from build123d import *

# Parameters (mm, degrees)
SKETCH1_W                      = 60
SKETCH1_H                      = 430.5
BASE_FLANGE1_DEPTH             = 4
EDGE_FLANGE1_STRIP_W           = 18
EDGE_FLANGE1_STRIP_H           = 4
EDGE_FLANGE1_STRIP_CUT_DEPTH   = 430.5
EDGE_FLANGE1_DEPTH             = 430.5
EDGE_FLANGE2_STRIP_W           = 18
EDGE_FLANGE2_STRIP_H           = 4
EDGE_FLANGE2_STRIP_CUT_DEPTH   = 55
EDGE_FLANGE2_STRIP_2_W         = 18
EDGE_FLANGE2_STRIP_2_H         = 4
EDGE_FLANGE2_STRIP_CUT_2_DEPTH = 55
EDGE_FLANGE2_STRIP_3_W         = 18
EDGE_FLANGE2_STRIP_3_H         = 4
EDGE_FLANGE2_STRIP_CUT_3_DEPTH = 55
EDGE_FLANGE2_STRIP_4_W         = 18
EDGE_FLANGE2_STRIP_4_H         = 4
EDGE_FLANGE2_STRIP_CUT_4_DEPTH = 55
EDGE_FLANGE2_DEPTH             = 55
EDGE_FLANGE2_BEND_DEPTH        = 55
EDGE_FLANGE2_BEND_2_DEPTH      = 55
EDGE_FLANGE2_BEND_3_DEPTH      = 55
SKETCH18_R                     = 4.6
EXTRUDE1_DEPTH                 = 440.643321341
SKETCH19_R                     = 4.6
EXTRUDE2_DEPTH                 = 4
SKETCH20_R                     = 4.6
EXTRUDE3_DEPTH                 = 4


# Sheet-metal steps are written as plain solids
with BuildPart() as part:
    # Sketch1 → Base-Flange1 (new body)
    with BuildSketch(Plane(origin=(0, 0, 0), x_dir=(1, 0, 0), z_dir=(0, 1, 0))):
        Rectangle(SKETCH1_W, SKETCH1_H)
    extrude(amount=BASE_FLANGE1_DEPTH)

    # Edge-Flange1 strip (across the edge) → Edge-Flange1 strip cut (cut)
    with BuildSketch(Plane(origin=(-30, 4, -215.25), x_dir=(1, 0, 0), z_dir=(0, 0, 1))):
        with Locations((-4, -2)):
            Rectangle(EDGE_FLANGE1_STRIP_W, EDGE_FLANGE1_STRIP_H)
    extrude(amount=EDGE_FLANGE1_STRIP_CUT_DEPTH, mode=Mode.SUBTRACT)

    # Edge-Flange1 section (across the edge) → Edge-Flange1 (add)
    with BuildSketch(Plane(origin=(-30, 4, -215.25), x_dir=(1, 0, 0), z_dir=(0, 0, 1))):
        with BuildLine():
            Line((0, 1), (0, 56))
            Line((0, 56), (4, 56))
            Line((4, 56), (4, 1))
            ThreePointArc((4, 1), (4.292893219, 0.292893219), (5, 0))
            Line((5, 0), (5, -4))
            ThreePointArc((5, -4), (1.464466094, -2.535533906), (0, 1))
        make_face()
    extrude(amount=EDGE_FLANGE1_DEPTH)

    # Edge-Flange2 strip (across the edge) → Edge-Flange2 strip cut (cut)
    with BuildSketch(Plane(origin=(-30, 5, 215.25), x_dir=(0, 0, -1), z_dir=(0, 1, 0))):
        with Locations((-4, -2)):
            Rectangle(EDGE_FLANGE2_STRIP_W, EDGE_FLANGE2_STRIP_H)
    extrude(amount=EDGE_FLANGE2_STRIP_CUT_DEPTH, mode=Mode.SUBTRACT)

    # Edge-Flange2 strip 2 (across the edge) → Edge-Flange2 strip cut 2 (cut)
    with BuildSketch(Plane(origin=(30, 0, 215.25), x_dir=(0, 0, -1), z_dir=(-1, 0, 0))):
        with Locations((-4, -2)):
            Rectangle(EDGE_FLANGE2_STRIP_2_W, EDGE_FLANGE2_STRIP_2_H)
    extrude(amount=EDGE_FLANGE2_STRIP_CUT_2_DEPTH, mode=Mode.SUBTRACT)

    # Edge-Flange2 strip 3 (across the edge) → Edge-Flange2 strip cut 3 (cut)
    with BuildSketch(Plane(origin=(-30, 60, -215.25), x_dir=(0, 0, 1), z_dir=(0, -1, 0))):
        with Locations((-4, -2)):
            Rectangle(EDGE_FLANGE2_STRIP_3_W, EDGE_FLANGE2_STRIP_3_H)
    extrude(amount=EDGE_FLANGE2_STRIP_CUT_3_DEPTH, mode=Mode.SUBTRACT)

    # Edge-Flange2 strip 4 (across the edge) → Edge-Flange2 strip cut 4 (cut)
    with BuildSketch(Plane(origin=(-25, 0, -215.25), x_dir=(0, 0, 1), z_dir=(1, 0, 0))):
        with Locations((-4, -2)):
            Rectangle(EDGE_FLANGE2_STRIP_4_W, EDGE_FLANGE2_STRIP_4_H)
    extrude(amount=EDGE_FLANGE2_STRIP_CUT_4_DEPTH, mode=Mode.SUBTRACT)

    # Edge-Flange2 section (across the edge) → Edge-Flange2 (add)
    with BuildSketch(Plane(origin=(-30, 5, 215.25), x_dir=(0, 0, -1), z_dir=(0, 1, 0))):
        with BuildLine():
            Line((0, 1), (0, 36))
            Line((0, 36), (4, 36))
            Line((4, 36), (4, 1))
            ThreePointArc((4, 1), (4.292893219, 0.292893219), (5, 0))
            Line((5, 0), (5, -4))
            ThreePointArc((5, -4), (1.464466094, -2.535533906), (0, 1))
        make_face()
    extrude(amount=EDGE_FLANGE2_DEPTH)

    # Edge-Flange2 section 2 (across the edge) → Edge-Flange2 bend (add)
    with BuildSketch(Plane(origin=(30, 0, 215.25), x_dir=(0, 0, -1), z_dir=(-1, 0, 0))):
        with BuildLine():
            Line((0, 1), (0, 36))
            Line((0, 36), (4, 36))
            Line((4, 36), (4, 1))
            ThreePointArc((4, 1), (4.292893219, 0.292893219), (5, 0))
            Line((5, 0), (5, -4))
            ThreePointArc((5, -4), (1.464466094, -2.535533906), (0, 1))
        make_face()
    extrude(amount=EDGE_FLANGE2_BEND_DEPTH)

    # Edge-Flange2 section 3 (across the edge) → Edge-Flange2 bend 2 (add)
    with BuildSketch(Plane(origin=(-30, 60, -215.25), x_dir=(0, 0, 1), z_dir=(0, -1, 0))):
        with BuildLine():
            Line((0, 1), (0, 36))
            Line((0, 36), (4, 36))
            Line((4, 36), (4, 1))
            ThreePointArc((4, 1), (4.292893219, 0.292893219), (5, 0))
            Line((5, 0), (5, -4))
            ThreePointArc((5, -4), (1.464466094, -2.535533906), (0, 1))
        make_face()
    extrude(amount=EDGE_FLANGE2_BEND_2_DEPTH)

    # Edge-Flange2 section 4 (across the edge) → Edge-Flange2 bend 3 (add)
    with BuildSketch(Plane(origin=(-25, 0, -215.25), x_dir=(0, 0, 1), z_dir=(1, 0, 0))):
        with BuildLine():
            Line((0, 1), (0, 36))
            Line((0, 36), (4, 36))
            Line((4, 36), (4, 1))
            ThreePointArc((4, 1), (4.292893219, 0.292893219), (5, 0))
            Line((5, 0), (5, -4))
            ThreePointArc((5, -4), (1.464466094, -2.535533906), (0, 1))
        make_face()
    extrude(amount=EDGE_FLANGE2_BEND_3_DEPTH)

    # Sketch18 → Extrude1 (cut, through all)
    with BuildSketch(Plane.XY.offset(215.25)):
        with Locations((-46, 47.5)):
            Circle(SKETCH18_R)
        with Locations((-46, 17.5)):
            Circle(SKETCH18_R)
        with Locations((-12.5, -16)):
            Circle(SKETCH18_R)
        with Locations((17.5, -16)):
            Circle(SKETCH18_R)
    extrude(amount=-EXTRUDE1_DEPTH, mode=Mode.SUBTRACT)

    # Sketch19 → Extrude2 (cut)
    with BuildSketch(Plane(origin=(-26, 0, 0), x_dir=(0, 0, -1), z_dir=(1, 0, 0))):
        with Locations(Location((-155.25, 35, 0), (0, 0, 90))):
            Circle(SKETCH19_R)
        with Locations(Location((135.25, 35, 0), (0, 0, 90))):
            Circle(SKETCH19_R)
    extrude(amount=-EXTRUDE2_DEPTH, mode=Mode.SUBTRACT)

    # Sketch20 → Extrude3 (cut)
    with BuildSketch(Plane(origin=(0, 4, 0), x_dir=(1, 0, 0), z_dir=(0, 1, 0))):
        with Locations(Location((5, 135.25, 0), (0, 0, 270))):
            Circle(SKETCH20_R)
        with Locations(Location((5, -155.25, 0), (0, 0, 270))):
            Circle(SKETCH20_R)
    extrude(amount=-EXTRUDE3_DEPTH, mode=Mode.SUBTRACT)


solid = part.part
Geometry: final body of the model. Coordinates: model frame, mm. A direction names the side the tool comes from. Round coordinates to 2 decimals unless told otherwise and drop trailing zeros. Loops run counter-clockwise (first coordinate to the right, second up) from the corner with the lowest first, then second, coordinate; pieces in that order, holes last. Notation, with made-up numbers: (48.25, 81) -> (74.25, 81) arc R27 ccw to (74.25, 117) -> close; hole circle Ø9 at (4.5, 28). An arc over 180 degrees is marked (long way). One line per question, with ' | ' between items. Start each with the question number.
1. Mould query, pull axis Z, two halves, no side actions, for faces 5 (the face through (3, -18, 215.25)), 6 (the face through (6.38, 2.03, 159.64)), 7 (the face through (-10.03, -12.12, -213.22)). Classes: pulls with the +Z half, pulls with the -Z half, needs draft (parallel to the pull), parting line crosses it, or undercut.
2. Contact query for flat-ended pins moving along their axis: pin 1 (8 mm diameter, centred on y = 36.5, z = 85, fed in from -X); pin 2 (14.5 mm diameter, centred on x = 5, z = 155.25, fed in from -Y); pin 3 (2.5 mm diameter, centred on x = -55.5, z = -213, fed in from -Y); pin 4 (7.5 mm diameter, centred on x = -46, y = 47.5, fed in from +Z). Output: stop coordinate, or through.
3. Line query: line 1 along Y through (x, z) = (-46, 213); line 2 along Z through (x, y) = (-23.5, -9.5); line 3 along X through (y, z) = (21.5, 109.5). Output: solid intervals per line, ascending. Write a range as [from, to].
4. Set-up query: faces 1 (the face through (-10.03, -12.12, 213.28)), 2 (the face through (2, 4, -3)), 3 (the face through (2, -19, -211.25)), 4 (the face through (-49, 32, 211.25)). Return all of +Z, -Z, +X, -X, +Y, -Y with unobstructed straight access to the full face (end or side cutting, diameter ignored); none if empty.
5. Section A-A on y = -16. Output: boundary loops of the cut face in (x, z).
6. Section C-C on y = 47.5. Output: boundary loops of the cut face in (x, z).
7. Section B-B on x = 5. Output: boundary loops of the cut face in (y, z), and give its area (3 significant figures).
8. Section D-D on z = -135.25. Output: boundary loops of the cut face in (x, y).
Returned:
1) face 5: pulls with the +Z half | face 6: undercut | face 7: needs draft
2) pin 1: stops at x = -30 | pin 2: stops at y = 0 | pin 3: stops at y = 5 | pin 4: passes through
3) line 1: y = [5, 12.9], [22.1, 42.9], [52.1, 60] | line 2: z = [-215.25, -211.25], [211.25, 215.25] | line 3: x = [-30, -26]
4) face 1: +Z, -Z | face 2: +Z, -Z, +X, +Y | face 3: +X, -X, -Y | face 4: -X, +Y, -Y
5) outline: (-25, -215.25) -> (-17.1, -215.25) -> (-17.1, -211.25) -> (-25, -211.25) -> close; (-25, 211.25) -> (-17.1, 211.25) -> (-17.1, 215.25) -> (-25, 215.25) -> close; (-7.9, -215.25) -> (12.9, -215.25) -> (12.9, -211.25) -> (-7.9, -211.25) -> close; (-7.9, 211.25) -> (12.9, 211.25) -> (12.9, 215.25) -> (-7.9, 215.25) -> close; (22.1, -215.25) -> (30, -215.25) -> (30, -211.25) -> (22.1, -211.25) -> close; (22.1, 211.25) -> (30, 211.25) -> (30, 215.25) -> (22.1, 215.25) -> close
6) outline: (-66, -215.25) -> (-50.6, -215.25) -> (-50.6, -211.25) -> (-66, -211.25) -> close; (-66, 211.25) -> (-50.6, 211.25) -> (-50.6, 215.25) -> (-66, 215.25) -> close; (-41.4, -215.25) -> (-31, -215.25) arc R5 ccw to (-26, -210.25) -> (-26, 210.25) arc R5 ccw to (-31, 215.25) -> (-41.4, 215.25) -> (-41.4, 211.25) -> (-31, 211.25) arc R1 cw to (-30, 210.25) -> (-30, -210.25) arc R1 cw to (-31, -211.25) -> (-41.4, -211.25) -> close
7) outline: (-36, -215.25) -> (-1, -215.25) arc R5 ccw to (4, -210.25) -> (4, -139.85) -> (0, -139.85) -> (0, -210.25) arc R1 cw to (-1, -211.25) -> (-36, -211.25) -> close; (-36, 211.25) -> (-1, 211.25) arc R1 cw to (0, 210.25) -> (0, 159.85) -> (4, 159.85) -> (4, 210.25) arc R5 ccw to (-1, 215.25) -> (-36, 215.25) -> close; (0, -130.65) -> (4, -130.65) -> (4, 150.65) -> (0, 150.65) -> close | area: 1,930 mm2
8) outline: (-30, 5) arc R5 ccw to (-25, 0) -> (0.4, 0) -> (0.4, 4) -> (-25, 4) arc R1 cw to (-26, 5) -> (-26, 30.4) -> (-30, 30.4) -> close; (-30, 39.6) -> (-26, 39.6) -> (-26, 60) -> (-30, 60) -> close; (9.6, 0) -> (30, 0) -> (30, 4) -> (9.6, 4) -> close
